For this review, use the dimensioned drawing (mm, ordinates from the lowest corner) and the shaded views. Give positions to 0.01 mm unless a question says otherwise; leave off trailing zeros. Write each loop counter-clockwise with the first axis right and the second up, starting at its lowest first coordinate (ties: lowest second). Pieces come first, ordered by that corner, then holes. Notation, with made-up numbers: M -0.5,18 L 43.5,18 A25 cw 43.5,33 Z; hole C 36.5,6.5 d8. An arc over 180 degrees is marked long. One line per item, written item: value. Start each with the question number.
Item 1: To check wall thickness, follow probe 1 along X at (y, z) = (2.25, 51.5); probe 2 along X at (y, z) = (1.2, 39); probe 3 along Z at (x, y) = (25.5, 0.35). State the ranges of each line that lie inside material, in increasing order.
Item 2: Consider section C-C, the plane z = 21.5. Write out the cut boundary in (x, y).
Item 3: Consider section D-D, the plane x = 41.5. Write out the cut boundary in (y, z).
Item 4: Consider section A-A, the plane y = 1.3. Write out the cut boundary in (x, z), and give its area (3 significant figures).
Item 5: Clearance check with flat-ended pins moving along their axes: pin 1 Ø1 at (x, y) = (44.5, 2) entering from -Z; pin 2 Ø0.8 at (x, y) = (6.5, 0.5) entering from +Z; pin 3 Ø0.8 at (y, z) = (1, 3) entering from +X. State where each tip first meets the part, or that it passes through.
Item 6: Consider section B-B, the plane x = 10.5. Write out the cut boundary in (y, z), and give its area (3 significant figures).
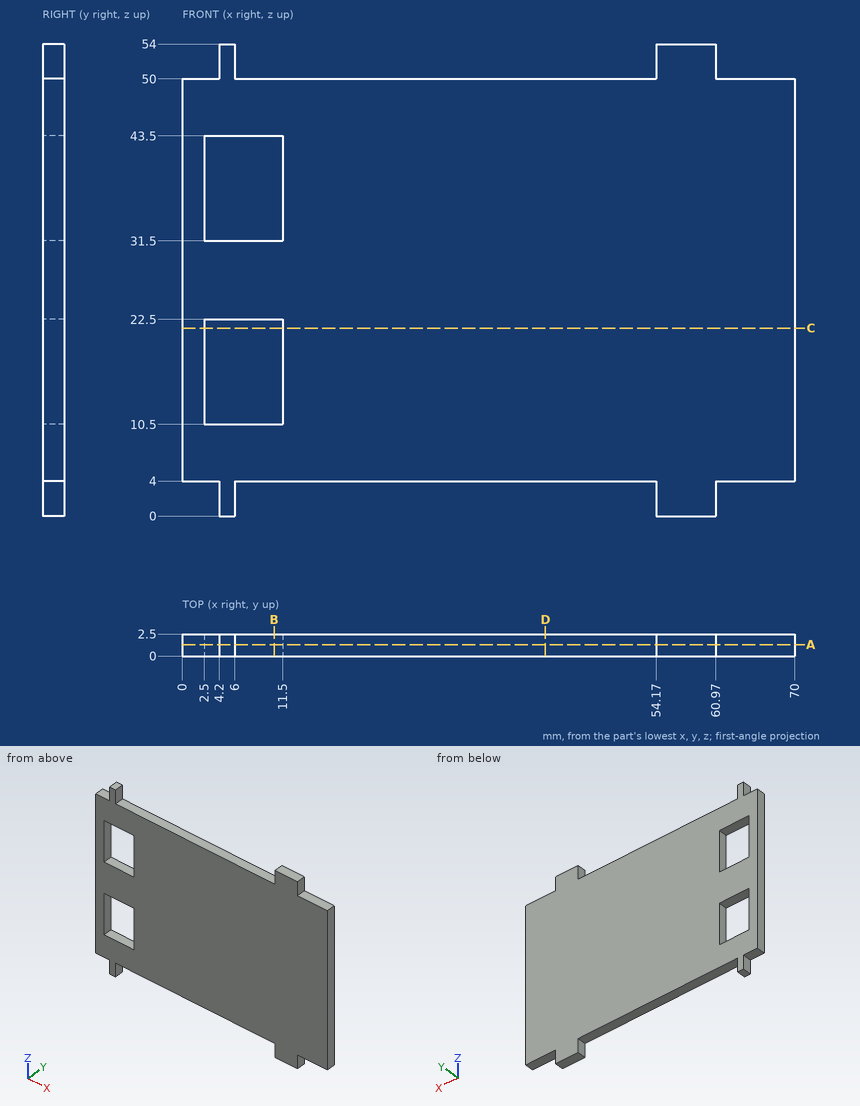
Model answer:
1. probe 1: x = 4.2 to 6, 54.17 to 60.97
1. probe 2: x = 0 to 2.5, 11.5 to 70
1. probe 3: z = 4 to 50
2. outline: M 0,0 L 2.5,0 L 2.5,2.5 L 0,2.5 Z; M 11.5,0 L 70,0 L 70,2.5 L 11.5,2.5 Z
3. outline: M 0,4 L 2.5,4 L 2.5,50 L 0,50 Z
4. outline: M 0,4 L 4.2,4 L 4.2,0 L 6,0 L 6,4 L 54.17,4 L 54.17,0 L 60.97,0 L 60.97,4 L 70,4 L 70,50 L 60.97,50 L 60.97,54 L 54.17,54 L 54.17,50 L 6,50 L 6,54 L 4.2,54 L 4.2,50 L 0,50 Z; hole M 2.5,10.5 L 11.5,10.5 L 11.5,22.5 L 2.5,22.5 Z; hole M 2.5,31.5 L 11.5,31.5 L 11.5,43.5 L 2.5,43.5 Z
4. area: 3,070 mm2
5. pin 1: stops at z = 4
5. pin 2: stops at z = 50
5. pin 3: stops at x = 60.97
6. outline: M 0,4 L 2.5,4 L 2.5,10.5 L 0,10.5 Z; M 0,22.5 L 2.5,22.5 L 2.5,31.5 L 0,31.5 Z; M 0,43.5 L 2.5,43.5 L 2.5,50 L 0,50 Z
6. area: 55.0 mm2
